Autodesk Inventor part; units mm, degrees
ref_plane "YZ Plane" through (0, 0, 0) normal (1, 0, 0) x (0, 1, 0)
ref_plane "XZ Plane" through (0, 0, 0) normal (0, 1, 0) x (-1, 0, 0)
ref_plane "XY Plane" through (0, 0, 0) normal (0, 0, 1) x (1, 0, 0)
sketch "Sketch1" plane through (0, 0, 0) normal (0, 1, 0) x (-1, 0, 0)
  line L0 (0, 0) -> (45, 0)
  line L1 (45, 0) -> (45, -83)
  line L2 (45, -83) -> (0, -83)
  line L3 (0, -83) -> (0, 0)
  circle A0 centre (39, -73) radius 2
  line L4 (22.5, 0) -> (22.5, -83)
  circle A1 centre (22.5, -43.5) radius 11.5
  circle A2 centre (38.1, -28) radius 1.5
  circle A3 centre (38, -59) radius 1.5
  circle A4 centre (6, -73) radius 2
  circle A5 centre (6.9, -28) radius 1.5
  circle A6 centre (7, -59) radius 1.5
  line L5 (45, -10) -> (0, -10)
  line L6 (6, -3.5) -> (11.525, -3.5)
  line L7 (11.525, -3.5) -> (11.525, -5)
  line L8 (11.525, -5) -> (6, -5)
  line L9 (6, -5) -> (6, -3.5)
  line L10 (6, -16.5) -> (11.525, -16.5)
  line L11 (11.525, -16.5) -> (11.525, -15)
  line L12 (11.525, -15) -> (6, -15)
  line L13 (6, -15) -> (6, -16.5)
  line L14 (39, -3.5) -> (33.475, -3.5)
  line L15 (33.475, -3.5) -> (33.475, -5)
  line L16 (33.475, -5) -> (39, -5)
  line L17 (39, -5) -> (39, -3.5)
  line L18 (39, -16.5) -> (33.475, -16.5)
  line L19 (33.475, -15) -> (39, -15)
  line L20 (39, -15) -> (39, -16.5)
  line L21 (33.475, -16.5) -> (33.475, -15)
  dimension "d0" = 45
  dimension "d1" = 83
  dimension "d2" = 10
  dimension "d3" = 6
  dimension "d9" = 4
  dimension "d13" = 45
  dimension "d14" = 24
  dimension "d15" = 31
  dimension "d16" = 31
  dimension "d17" = 15.5
  dimension "d18" = 23
  dimension "d19" = 3
  dimension "d20" = 3
  dimension "d22" = 20
  dimension "d23" = 6
  dimension "d24" = 10
  dimension "d25" = 1.5
extrude "Extrusion2" add sketch "Sketch1" along normal blind 1 contours L0 L4 L5 L3 | L0 L1 L5 L4 | L5 L4 A1 L2 L3 | L5 L1 L2 L4 A1
equation "\"d13\" = d0"
properties part number "Platte1"
CAD build for the part. Positions are in the model's coordinates, mm. Coordinates: 2 decimals unless noted, no trailing zeros. Order: outer loops, then holes, each group sorted by start corner. A loop starts at its lowest first (then second) coordinate and runs counter-clockwise, first axis right, second up. Notation, with made-up numbers: M 8.5,0 L 41.5,0 A24 cw 41.5,27 Z; hole C 40.25,4 d9. An arc over 180 degrees is marked long. Answer as CSV lines item,"result".
1) Cut at D-D (y = 0.75). Give the number of separate pieces and of enclosed holes in the cut face, then the cut area to 3 significant figures.
Verdict:
separate pieces,"1"
enclosed holes,"11"
area,"3,230 mm2"
2) Flat gauge pins, fed straight in: P1, Ø1, axis at x = -39.5, z = -23, coming from the -Y side; P2, Ø20.5, axis at x = -22.5, z = -43.5, coming from the -Y side. Where does each tip first touch, or does it go through?
Verdict:
P1,"y = 0"
P2,"through"
3) Cut at A-A (z = -59). List the corners of the cut face in (x, y), then the cut area to 3 significant figures.
Verdict:
outline,"M -45,0 L -39.5,0 L -39.5,1 L -45,1 Z; M -36.5,0 L -8.5,0 L -8.5,1 L -36.5,1 Z; M -5.5,0 L 0,0 L 0,1 L -5.5,1 Z"
area,"39.0 mm2"
4) Drill centre lines: L1, parallel to X at y = 0.6, z = -43.5; L2, parallel to Z at x = -6.9, y = 0.75; L3, parallel to Z at x = -37.5, y = 0.9. Where is each one in solid material? Low to high. Write a range as from..to.
Verdict:
L1,"-45..-34, -11..0"
L2,"-83..-74.79, -71.21..-60.5, -57.5..-29.5, -26.5..-16.5, -15..-5, -3.5..0"
L3,"-83..-74.32, -71.68..-60.41, -57.59..-29.37, -26.63..-16.5, -15..-5, -3.5..0"
5) Mould opens along X. For faces 1 (the flat face through (-22.2, 0, -31.7)), 2 (the cylindrical face through (-5.74, 0.493, -74.983)) say: released by +X, released by -X, zero draft, split by the parting line, or undercut.
Verdict:
face 1,"zero draft"
face 2,"undercut"
6) Cut at B-B (z = -43.5). List the corners of the cut face in (x, y).
Verdict:
outline,"M -45,0 L -34,0 L -34,1 L -45,1 Z; M -11,0 L 0,0 L 0,1 L -11,1 Z"
7) Cut at C-C (x = -22.5). List the corners of the cut face in (y, z), then the cut area to 3 significant figures.
Verdict:
outline,"M 0,-83 L 1,-83 L 1,-55 L 0,-55 Z; M 0,-32 L 1,-32 L 1,0 L 0,0 Z"
area,"60.0 mm2"
